Model file for the job. Use its own axes, mm. A direction names the side the tool comes from. Coordinates: 2 decimals unless noted, no trailing zeros. Write each loop counter-clockwise with the first axis right and the second up, starting at its lowest first coordinate (ties: lowest second). Pieces come first, ordered by that corner, then holes. Notation, with made-up numbers: (32, 37.25) - (57, 37.25) arc R26 cw to (57, 57.25) - close; hole circle Ø3 at (21.5, -17.75). An arc over 180 degrees is marked (long way). Put each result on its own line as item: value. Start each with the question number.
1. Pull direction X, two halves, no side cores. Call faces 1 (the face through (4.119, -18.548, -8.57)), 2 (the face through (4.259, -0.445, -8.619)), 3 (the face through (0, 4, 0)): released by +X, released by -X, zero draft, split by the parting line, or undercut.
2. Drill centre lines: L1, parallel to Y at x = 0, z = -12.5; L2, parallel to Z at x = 0, y = -16; L3, parallel to X at y = -16.5, z = -8.5. Where is each one in solid material? Low to high. Write a range as from..to.
3. Saw through at A-A, the plane x = 0. Write the cut outline in (y, z), plus the area to 3 significant figures.
4. Saw through at B-B, the plane z = -10. Write the cut outline in (x, y).
5. Which spindle directions (+Z, -Z, +X, -X, +Y, -Y) get a long thin tool onto all of the face, cutting with end or side? Do faces 4 (the face through (0, 4, -17)), 5 (the face through (-11, 16, -13.5)). Say none if no direction does.
6. Drop flat-ended pins along their axis: P1, Ø2, axis at y = 13, z = -5.5, coming from the +X side; P2, Ø2, axis at x = 4.5, z = -7, coming from the +Y side; P3, Ø7, axis at x = 0, z = -8.5, coming from the +Y side. Give the stop position or say it passes through.
7. Saw through at C-C, the plane z = -2.25. Write the cut outline in (x, y), plus the area to 3 significant figures.
8. Saw through at D-D, the plane z = -6.5. Write the cut outline in (x, y), plus the area to 3 significant figures.
Autodesk Inventor part; units mm, degrees
ref_plane "Work Plane1" through (0, 20, 0) normal (0, 1, 0) x (-1, 0, 0)
ref_plane "YZ Plane" through (0, 0, 0) normal (1, 0, 0) x (0, 1, 0)
ref_plane "XY Plane" through (0, 0, 0) normal (0, 0, 1) x (1, 0, 0)
sketch "Sketch1" plane through (0, 0, 0) normal (0, 1, 0) x (-1, 0, 0)
  line L0 (0, 0) -> (21.5, 0)
  line L1 (21.5, 0) -> (21.5, -3.5)
  line L2 (21.5, -3.5) -> (19, -3.5)
  line L3 (19, -3.5) -> (19, -13.5)
  line L4 (19, -13.5) -> (21.5, -13.5)
  line L5 (21.5, -13.5) -> (21.5, -17)
  line L6 (21.5, -17) -> (0, -17)
  line L7 (0, -17) -> (0, 0)
  dimension "d1" = 3.5
  dimension "d2" = 3.5
  dimension "d3" = 17
  dimension "d4" = 38
  dimension "d5" = 43
revolve "Revolution1" add sketch "Sketch1" angle 360 about axis through (0, 0, -17) along (0, 0, 1)
sketch "Sketch2" plane through (0, 0, 0) normal (0, 0, 1) x (1, 0, 0)
  point P0 (0, 0)
  point P1 (0, -6)
  dimension "d14" = 6
hole "Hole1" at (0, -6, 0) direction (0, 0, -1) diameter 14 depth 17
fillet "Fillet1" radius 1 2 edges at (21.5, 0, 0) (21.5, 0, -17)
ref_plane "Work Plane1" through (0, 20, 0) normal (0, 1, 0) x (-1, 0, 0)
sketch "Sketch4" plane through (0, 20, 0) normal (0, 1, 0) x (-1, 0, 0)
  circle A0 centre (0, -8.5) radius 3
  line L0 (19, -13.5) -> (19, -3.5)
  point P0 (0, 0)
  point P1 (19, -8.5)
  dimension "d17" = 6
extrude "Extrusion1" cut sketch "Sketch4" against normal through all
properties part number "204"
Final values:
1. face 1: split by the parting line
1. face 2: undercut
1. face 3: zero draft
2. L1: y = -19..-13, 1..19
2. L2: z = -17..-11.5, -5.5..0
2. L3: x = -9.42..-3, 3..9.42
3. outline: (-21.5, -16) arc R1 ccw to (-20.5, -17) - (-13, -17) - (-13, -11.5) - (-19, -11.5) - (-19, -13.5) - (-21.5, -13.5) - close; (-21.5, -3.5) - (-19, -3.5) - (-19, -5.5) - (-13, -5.5) - (-13, 0) - (-20.5, 0) arc R1 ccw to (-21.5, -1) - close; (1, -17) - (20.5, -17) arc R1 ccw to (21.5, -16) - (21.5, -13.5) - (19, -13.5) - (19, -11.5) - (1, -11.5) - close; (1, -5.5) - (19, -5.5) - (19, -3.5) - (21.5, -3.5) - (21.5, -1) arc R1 ccw to (20.5, 0) - (1, 0) - close
3. area: 298 mm²
4. outline: (-2.6, -18.82) - (-2.6, -12.5) arc R7 cw to (-2.6, 0.5) - (-2.6, 18.82) arc R19 ccw to start; (2.6, -18.82) arc R19 ccw to (2.6, 18.82) - (2.6, 0.5) arc R7 cw to (2.6, -12.5) - close
5. face 4: -Z, +X, -X, +Y, -Y
5. face 5: none
6. P1: stops at x = 14.73
6. P2: stops at y = 18.67
6. P3: stops at y = 19
7. outline: circle Ø43 at (0, 0); hole circle Ø14 at (0, -6)
7. area: 1,300 mm²
8. outline: (-2.24, -18.87) - (-2.24, -12.63) arc R7 cw to (-2.24, 0.63) - (-2.24, 18.87) arc R19 ccw to start; (2.24, -18.87) arc R19 ccw to (2.24, 18.87) - (2.24, 0.63) arc R7 cw to (2.24, -12.63) - close
8. area: 872 mm²
